Geometry: see drawing. Coordinates: mm, zero at the bounding-box minimum. Coordinates: 2 decimals unless noted, no trailing zeros. Write each loop counter-clockwise with the first axis right and the second up, starting at its lowest first coordinate (ties: lowest second). Pieces come first, ordered by that corner, then holes. Notation, with made-up numbers: M 57.5,82.5 L 100.5,82.5 A18 ccw 100.5,97.5 Z; hole C 82,17 d2. An arc over 180 degrees is marked long. One line per item, written item: value. Start each with the question number.
Item 1: Mould query, pull axis X, two halves, no side actions, for the marked faces 1 and 2. Classes: released by +X, released by -X, zero draft, split by the parting line, or undercut.
Item 2: Cut plane C-C, the plane z = 1. Output: boundary loops of the cut face in (x, y) (3 decimals).
Item 3: Cut plane A-A, the plane y = 0.15. Output: boundary loops of the cut face in (x, z) (1 decimal), then the cut area to 3 significant figures.
Item 4: Cut plane B-B, the plane z = 7. Output: boundary loops of the cut face in (x, y) (3 decimals).
Item 5: Cut plane D-D, the plane z = 3.75. State how many separate pieces and enclosed holes the cut face has, then the cut area to 3 significant figures.
Item 6: Ray query, L1, parallel to Z at x = 20, y = 0.4 (1 decimal); L2, parallel to X at y = 0.1, z = 3.75 (1 decimal); L3, parallel to X at y = 0.4, z = 11 (3 decimals). Return the intervals inside material, ascending. Write a range as from..to.
Item 7: Pin query (flat end, axial travel): P1, Ø1.8, axis at x = 5.46, z = 9.6, coming from the -Y side; P2, Ø2, axis at x = 13, z = 3.5, coming from the +Y side. Return the tip coordinate at first contact, or that it passes through.
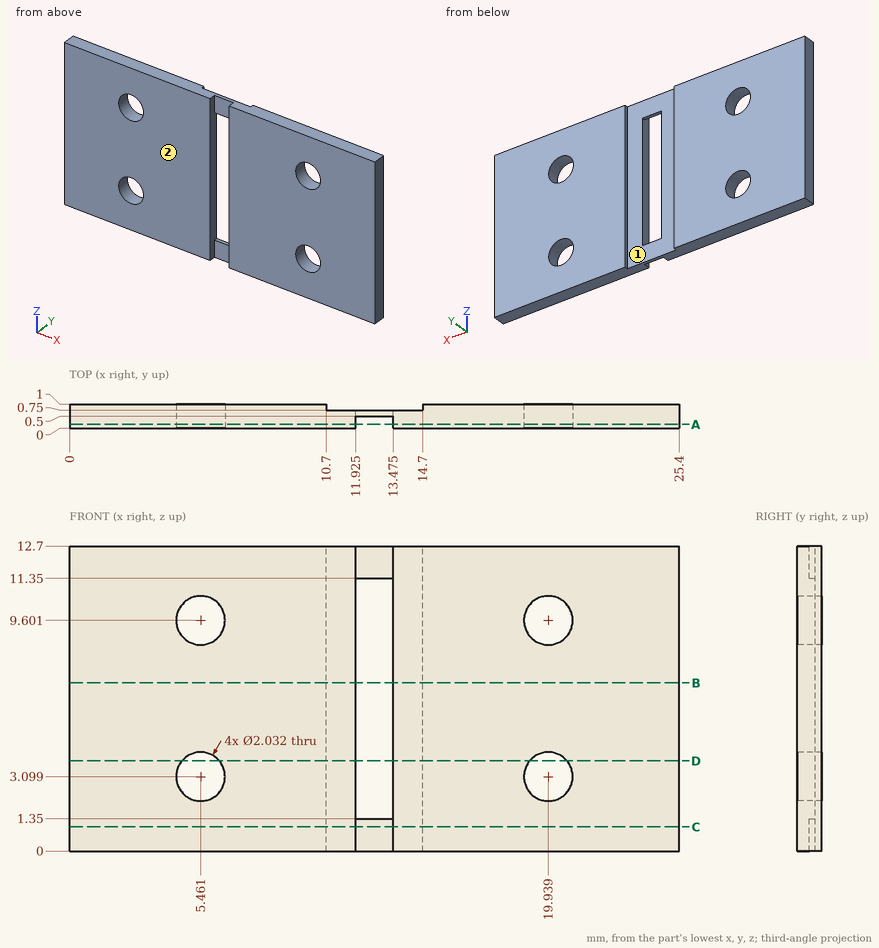
From the geometry:
1. face 1: undercut
1. face 2: zero draft
2. outline: M 0,0 L 11.925,0 L 11.925,0.5 L 13.475,0.5 L 13.475,0 L 25.4,0 L 25.4,1 L 14.7,1 L 14.7,0.75 L 10.7,0.75 L 10.7,1 L 0,1 Z
3. outline: M 0,0 L 11.9,0 L 11.9,12.7 L 0,12.7 Z; M 13.5,0 L 25.4,0 L 25.4,12.7 L 13.5,12.7 Z; hole C 5.5,3.1 d2; hole C 5.5,9.6 d2; hole C 19.9,3.1 d2; hole C 19.9,9.6 d2
3. area: 290 mm²
4. outline: M 0,0 L 11.925,0 L 11.925,0.75 L 10.7,0.75 L 10.7,1 L 0,1 Z; M 13.475,0 L 25.4,0 L 25.4,1 L 14.7,1 L 14.7,0.75 L 13.475,0.75 Z
5. separate pieces: 4
5. enclosed holes: 0
5. area: 20.1 mm²
6. L1: z = 0..2.1, 4.1..8.6, 10.6..12.7
6. L2: x = 0..4.7, 6.2..11.9, 13.5..19.2, 20.7..25.4
6. L3: x = 0..11.925, 13.475..25.4
7. P1: passes through
7. P2: stops at y = 0.75
